Could you check a few things on this model? Use its own coordinates, in mm. Face numbers are marked on the shaded views. A direction names the side the tool comes from. Coordinates: 2 decimals unless noted, no trailing zeros. Loops run counter-clockwise (first coordinate to the right, second up) from the corner with the lowest first, then second, coordinate; pieces in that order, holes last.
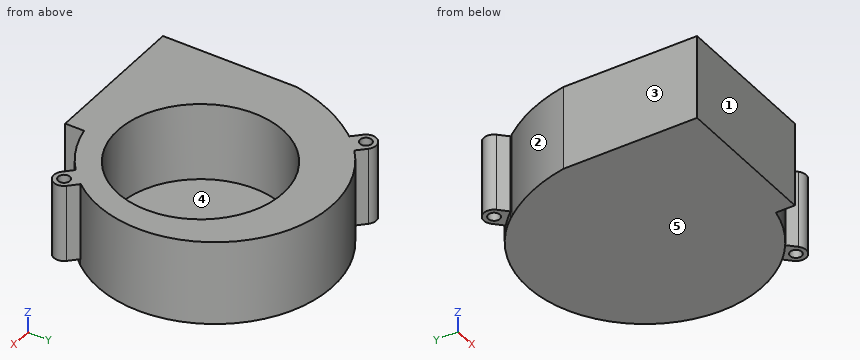
from build123d import *

# Parameters (mm, degrees)
F0_R     = 32
F0_R_2   = 2.25
F1_DEPTH = 30
F2_DEPTH = 2.7


with BuildPart() as f1:
    # F0 (on Top) → F1 (new body)
    with BuildSketch(Plane.XY):
        with BuildLine():
            Line((-48.5, 0), (-48.5, -51.8))
            Line((-48.5, -51.8), (9.5, -51.8))
            Line((9.5, -51.8), (9.5, -44.4971909226))
            ThreePointArc((9.5, -44.4971909226), (19.9487496546, -40.8937328599), (29.2203638041, -34.8772180536))
            ThreePointArc((29.2203638041, -34.8772180536), (32.173358544, -32.173358544), (34.8772180536, -29.2203638041))
            ThreePointArc((34.8772180536, -29.2203638041), (32.173358544, 32.173358544), (-29.2203638041, 34.8772180536))
            ThreePointArc((-29.2203638041, 34.8772180536), (-32.173358544, 32.173358544), (-34.8772180536, 29.2203638041))
            ThreePointArc((-34.8772180536, 29.2203638041), (-35.2558555468, 28.7623825449), (-35.6284796081, 28.2994954162))
            ThreePointArc((-35.6284796081, 28.2994954162), (-43.8019044029, 14.9400934365), (-48.5, 0))
        make_face()
        with Locations((3.25, -3.5)):
            Circle(F0_R, mode=Mode.SUBTRACT)
        with BuildLine():
            ThreePointArc((34.8772180536, -29.2203638041), (32.173358544, -32.173358544), (29.2203638041, -34.8772180536))
            Line((29.2203638041, -34.8772180536), (32.5269119346, -38.1837661841))
            ThreePointArc((32.5269119346, -38.1837661841), (38.1837661841, -38.1837661841), (38.1837661841, -32.5269119346))
            Line((38.1837661841, -32.5269119346), (34.8772180536, -29.2203638041))
        make_face()
        with Locations((35.3553390593, -35.3553390593)):
            Circle(F0_R_2, mode=Mode.SUBTRACT)
        with BuildLine():
            Line((-38.1837661841, 32.5269119346), (-34.8772180536, 29.2203638041))
            ThreePointArc((-34.8772180536, 29.2203638041), (-32.173358544, 32.173358544), (-29.2203638041, 34.8772180536))
            Line((-29.2203638041, 34.8772180536), (-32.5269119346, 38.1837661841))
            ThreePointArc((-32.5269119346, 38.1837661841), (-38.1837661841, 38.1837661841), (-38.1837661841, 32.5269119346))
        make_face()
        with Locations((-35.3553390593, 35.3553390593)):
            Circle(F0_R_2, mode=Mode.SUBTRACT)
    extrude(amount=F1_DEPTH)

    # F0 (on Top) → F2 (join)
    with BuildSketch(Plane.XY):
        with BuildLine():
            Line((-48.5, 0), (-48.5, -51.8))
            Line((-48.5, -51.8), (9.5, -51.8))
            Line((9.5, -51.8), (9.5, -44.4971909226))
            ThreePointArc((9.5, -44.4971909226), (19.9487496546, -40.8937328599), (29.2203638041, -34.8772180536))
            ThreePointArc((29.2203638041, -34.8772180536), (32.173358544, -32.173358544), (34.8772180536, -29.2203638041))
            ThreePointArc((34.8772180536, -29.2203638041), (32.173358544, 32.173358544), (-29.2203638041, 34.8772180536))
            ThreePointArc((-29.2203638041, 34.8772180536), (-32.173358544, 32.173358544), (-34.8772180536, 29.2203638041))
            ThreePointArc((-34.8772180536, 29.2203638041), (-35.2558555468, 28.7623825449), (-35.6284796081, 28.2994954162))
            ThreePointArc((-35.6284796081, 28.2994954162), (-43.8019044029, 14.9400934365), (-48.5, 0))
        make_face()
        with Locations((3.25, -3.5)):
            Circle(F0_R, mode=Mode.SUBTRACT)
        with Locations((3.25, -3.5)):
            Circle(F0_R)
    extrude(amount=-F2_DEPTH)


solid = f1.part
(1) Imagine slicing it at B-B, the plane z = 25. Write out the boundary of the cut face in (x, y), and give its area (3 significant figures).
Answers:
outline: (-48.5, -51.8) - (9.5, -51.8) - (9.5, -44.5) arc R45.5 ccw to (29.22, -34.88) - (32.53, -38.18) arc R4 ccw to (38.18, -32.53) - (34.88, -29.22) arc R45.5 ccw to (-29.22, 34.88) - (-32.53, 38.18) arc R4 ccw to (-38.18, 32.53) - (-34.88, 29.22) arc R45.5 ccw to (-35.63, 28.3) arc R64.24 ccw to (-48.5, 0) - close; hole circle Ø4.5 at (-35.36, 35.36); hole circle Ø64 at (3.25, -3.5); hole circle Ø4.5 at (35.36, -35.36)
area: 4,360 mm2
(2) We'd pull the mould along Y, two halves only. Please class the marked faces 1, 2 and 3: +Y half, -Y half, draft (parallel to the pull), parting line (faces both ways), or undercut.
Answers:
face 1: -Y half
face 2: undercut
face 3: draft
(3) Imagine slicing it at C-C, the plane y = -3.5. Write out the boundary of the cut face in (x, z).
Answers:
outline: (-48.5, -2.7) - (45.37, -2.7) - (45.37, 30) - (35.25, 30) - (35.25, 0) - (-28.75, 0) - (-28.75, 30) - (-48.5, 30) - close
(4) Which directions (+Z, -Z, +X, -X, +Y, -Y) give clear straight access to the entire face, cutting with the end or side of a thin tool? Please do the marked faces 4 and 5.
Answers:
face 4: +Z
face 5: -Z, +X, -X, +Y, -Y
(5) I need wall thicknesses on probe 1 along X at (y, z) = (3, 22); probe 2 along Y at (x, z) = (28, 16.5); probe 3 along Z at (x, y) = (33, 8). Which ranges of each line are inside material? Lowest first, please.
Answers:
probe 1: x = -47.87 to -28.08, 34.58 to 45.4
probe 2: y = -35.86 to -23.78, 16.78 to 35.86
probe 3: z = -2.7 to 0
(6) For pin 1 (5 mm diameter, centred on x = -34, y = 37, fed in from -Z); pin 2 (3 mm diameter, centred on x = -12, y = -15.5, fed in from +Z); pin 3 (2 mm diameter, centred on y = -24.5, z = 15.5, fed in from +X), each with a flat end and sliding along its axis, tell me the tip position at first contact or that it passes through.
Answers:
pin 1: stops at z = 0
pin 2: stops at z = 0
pin 3: stops at x = 38.96
(7) Imagine slicing it at A-A, the plane x = -13. Write out the boundary of the cut face in (y, z), and give its area (3 significant figures).
Answers:
outline: (-51.8, -2.7) - (43.6, -2.7) - (43.6, 30) - (24.07, 30) - (24.07, 0) - (-31.07, 0) - (-31.07, 30) - (-51.8, 30) - close
area: 1,470 mm2
